The model under review builds one solid part; all positions refer to its coordinate system, in mm. Coordinates: 2 decimals unless noted, no trailing zeros. Order: outer loops, then holes, each group sorted by start corner. A loop starts at its lowest first (then second) coordinate and runs counter-clockwise, first axis right, second up.
```python
from build123d import *

# Parameters (mm, degrees)
BOSS_EXTRUDE1_DEPTH   = 12
SKETCH3_R             = 3.6
CUT_EXTRUDE2_DEPTH    = 13
M5X0_8_TAPPED_HOLE1_D = 4.2


with BuildPart() as part:
    # Sketch1 → Boss-Extrude1 (new body)
    with BuildSketch(Plane.XY):
        with BuildLine():
            Line((39.84, -10), (-39.84, -10))
            ThreePointArc((-39.84, -10), (-42.215878785, -9.015878785), (-43.2, -6.64))
            Line((-43.2, -6.64), (-43.2, 6.64))
            ThreePointArc((-43.2, 6.64), (-42.215878785, 9.015878785), (-39.84, 10))
            Line((-39.84, 10), (39.84, 10))
            ThreePointArc((39.84, 10), (42.215878785, 9.015878785), (43.2, 6.64))
            Line((43.2, 6.64), (43.2, -6.64))
            ThreePointArc((43.2, -6.64), (42.215878785, -9.015878785), (39.84, -10))
        make_face()
    extrude(amount=BOSS_EXTRUDE1_DEPTH)

    # Sketch3 → Cut-Extrude2 (cut, through all)
    with BuildSketch(Plane.XY.offset(12)):
        with Locations((-30, 0)):
            Circle(SKETCH3_R)
        with Locations((30, 0)):
            Circle(SKETCH3_R)
        Circle(SKETCH3_R)
    extrude(amount=-CUT_EXTRUDE2_DEPTH, mode=Mode.SUBTRACT)

    # M5x0.8 Tapped Hole1 (through all)
    with Locations(Plane.XY.offset(12)):
        with Locations((-20, 0), (20, 0)):
            Hole(M5X0_8_TAPPED_HOLE1_D / 2)


solid = part.part
```
(1) We need section B-B, the plane x = 20. Write out the cut boundary in (y, z), and give its area (3 significant figures).
A:
outline: (-10, 0) - (-2.1, 0) - (-2.1, 12) - (-10, 12) - close; (2.1, 0) - (10, 0) - (10, 12) - (2.1, 12) - close
area: 190 mm2
(2) For pin 1 Ø4 at (x, y) = (-20, 0) entering from +Z, flat-tipped, find the tip position at first contact; note if it passes through.
A:
pin 1: passes through
(3) We need section A-A, the plane y = 0. Write out the cut boundary in (x, z).
A:
outline: (-43.2, 0) - (-33.6, 0) - (-33.6, 12) - (-43.2, 12) - close; (-26.4, 0) - (-22.1, 0) - (-22.1, 12) - (-26.4, 12) - close; (-17.9, 0) - (-3.6, 0) - (-3.6, 12) - (-17.9, 12) - close; (3.6, 0) - (17.9, 0) - (17.9, 12) - (3.6, 12) - close; (22.1, 0) - (26.4, 0) - (26.4, 12) - (22.1, 12) - close; (33.6, 0) - (43.2, 0) - (43.2, 12) - (33.6, 12) - close
(4) Wall thickness on probe 1 along Y at (x, z) = (20, 6); probe 2 along Y at (x, z) = (-30, 8); probe 3 along X at (y, z) = (3, 2.5): over which ranges is each line inside the solid? List them lowest first.
A:
probe 1: y = -10 to -2.1, 2.1 to 10
probe 2: y = -10 to -3.6, 3.6 to 10
probe 3: x = -43.2 to -31.99, -28.01 to -1.99, 1.99 to 28.01, 31.99 to 43.2
(5) We need section D-D, the plane x = 30. Write out the cut boundary in (y, z), and give its area (3 significant figures).
A:
outline: (-10, 0) - (-3.6, 0) - (-3.6, 12) - (-10, 12) - close; (3.6, 0) - (10, 0) - (10, 12) - (3.6, 12) - close
area: 154 mm2
(6) Draft analysis for pull direction Y (two halves, no side actions). For faces 1 (the face through (-42.24, 8.99, 5.92)), 2 (the face through (1, -10, 6)), 3 (the face through (3.434, 1.081, 6.084)), state which applies: released by +Y, released by -Y, zero draft, split by the parting line, or undercut.
A:
face 1: released by +Y
face 2: released by -Y
face 3: undercut
(7) We need section C-C, the plane z = 1.5. Write out the cut boundary in (x, y).
A:
outline: (-43.2, -6.64) arc R3.36 ccw to (-39.84, -10) - (39.84, -10) arc R3.36 ccw to (43.2, -6.64) - (43.2, 6.64) arc R3.36 ccw to (39.84, 10) - (-39.84, 10) arc R3.36 ccw to (-43.2, 6.64) - close; hole circle Ø7.2 at (-30, 0); hole circle Ø4.2 at (-20, 0); hole circle Ø7.2 at (0, 0); hole circle Ø4.2 at (20, 0); hole circle Ø7.2 at (30, 0)
